```python
from build123d import *

# Parameters (mm, degrees)
F0_R     = 26
F0_W     = 14.36842
F0_H     = 5.710526
F1_DEPTH = 20
F0_R_2   = 29
F2_DEPTH = 4
F3_SIZE  = 3


with BuildPart() as f1:
    # F0 (on Top) → F1 (new body)
    with BuildSketch(Plane.XY):
        Circle(F0_R)
        Rectangle(F0_W, F0_H, mode=Mode.SUBTRACT)
        Rectangle(F0_W, F0_H)
    extrude(amount=F1_DEPTH)

    # F0 (on Top) → F2 (join)
    with BuildSketch(Plane.XY):
        Circle(F0_R_2)
        Circle(F0_R, mode=Mode.SUBTRACT)
    extrude(amount=F2_DEPTH)

    # F3
    f3_edges = [f1.edges().sort_by_distance(p)[0] for p in [
        (-26, 0, 20),
    ]]
    chamfer(f3_edges, length=F3_SIZE)


solid = f1.part
```
Work out the finished part from the listing and answer in its coordinate system (mm). A direction names the side the tool comes from. Give positions to 0.01 mm unless a question says otherwise; leave off trailing zeros. Write each loop counter-clockwise with the first axis right and the second up, starting at its lowest first coordinate (ties: lowest second). Pieces come first, ordered by that corner, then holes. Notation, with made-up numbers: (-36.75, -2) -> (-8.75, -2) arc R26 ccw to (-8.75, 31) -> close; hole circle Ø3 at (33, 70.5). An arc over 180 degrees is marked (long way). Write item = value, one per line.
Q1. A tool of negligible diameter and unlimited length cuts with its end or side. For faces 1 (the flat face through (0, 0, 0)), 2 (the cylindrical face through (-20.633, -15.821, 10.409)), from which of +Z, -Z, +X, -X, +Y, -Y can it reach the whole face along a straight path? Write none if from no direction.
Computed values:
face_1 = -Z, +X, -X, +Y, -Y
face_2 = +Z
Q2. Consider line 1 along X through (y, z) = (-0.5, 11.5); line 2 along Z through (x, y) = (10.5, 25.5); line 3 along Y through (x, z) = (24.5, 3.75). Determine where each line is inside the solid, lowest interval first.
Computed values:
line_1 = -26 to 26
line_2 = 0 to 4
line_3 = -15.52 to 15.52
Q3. Section A-A on y = 0 is taken. Determine the outline of the cut face in (x, z).
Computed values:
outline = (-29, 0) -> (29, 0) -> (29, 4) -> (26, 4) -> (26, 17) -> (23, 20) -> (-23, 20) -> (-26, 17) -> (-26, 4) -> (-29, 4) -> close
Q4. Section C-C on z = 12.5 is taken. Determine the outline of the cut face in (x, y), and give its area (3 significant figures).
Computed values:
outline = circle Ø52 at (0, 0)
area = 2,120 mm^2
Q5. Flat-ended cylindrical pins translate along their axes: pin 1 Ø10 at (x, z) = (2.5, 4.5) entering from -Y; pin 2 Ø1.5 at (x, y) = (17, -17) entering from +Z; pin 3 Ø4 at (x, z) = (-12, 13.5) entering from -Y. Find the tip coordinate at first contact, or state that the pin passes through.
Computed values:
pin_1 = -29
pin_2 = 19.71
pin_3 = -24
